Can you work these out from the model? Positions are in its coordinate system, mm. Face numbers are marked on the shaded views. A direction names the side the tool comes from. Give positions to 0.01 mm unless a question says otherwise; leave off trailing zeros. Write each loop counter-clockwise with the first axis right and the second up, starting at its lowest first coordinate (ties: lowest second). Pieces come first, ordered by that corner, then holes. Notation, with made-up numbers: (11.25, 77.25) - (69.25, 77.25) arc R15 cw to (69.25, 87.25) - close; hole circle Ø8 at (58, 0). An arc over 180 degrees is marked (long way). Use a Markdown table: item, result. Add a question column.
```python
from build123d import *

# Parameters (mm, degrees)
F2_W     = 460
F2_H     = 460
F2_W_2   = 420
F2_H_2   = 420
F3_DEPTH = 460
F4_R     = 5
F5_R     = 5


# Not quite as in the source:
# - the program builds the solid bodies; features that only make, move or delete a surface that nothing else refers to are left out


with BuildPart() as f3:
    # F2 (on Top) → F3 (new body)
    with BuildSketch(Plane.XY):
        Rectangle(F2_W, F2_H)
        Rectangle(F2_W_2, F2_H_2, mode=Mode.SUBTRACT)
    extrude(amount=F3_DEPTH)

    # F4
    f4_edges = [f3.edges().sort_by_distance(p)[0] for p in [
        (-230, 230, 230),
    ]]
    fillet(f4_edges, radius=F4_R)

    # F5
    f5_edges = [f3.edges().sort_by_distance(p)[0] for p in [
        (-230, -2.5, 460),
    ]]
    fillet(f5_edges, radius=F5_R)


solid = f3.part
```
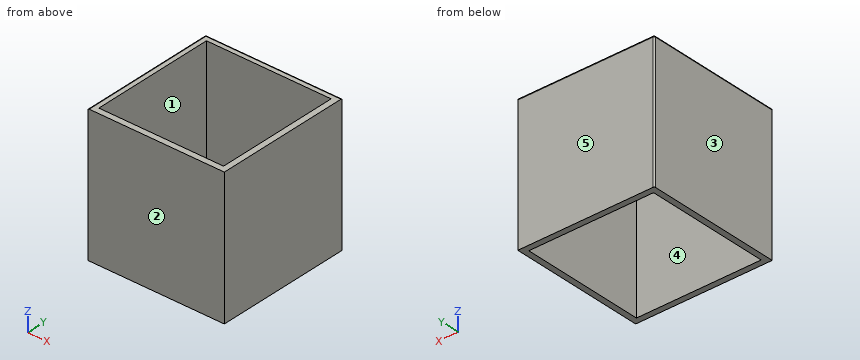
Q1. On a 3-axis mill with a long thin cutter (end or side, diameter ignored), from which of +Z, -Z, +X, -X, +Y, -Y can I reach the whole of each face in a straight line? I mean the marked faces 4 and 5. Say none if no direction works.
Q2. Suppose I cut it at C-C (y = -157.5). Please give me the cut outline in (x, z).
Q3. If I drill on probe 1 along Y at (x, z) = (-157.5, 179), over which ranges is the centre line in solid material (lowest first)? Write a range as [from, to].
Q4. Suppose I cut it at B-B (x = 30). Please give me the cut outline in (y, z), and give its area (3 significant figures).
Q5. If we mould it in two halves opening along X, with no side actions, what happens to the marked faces 1, 2 and 3? For each: released by +X, released by -X, zero draft, split by the parting line, or undercut.
Q6. Suppose I cut it at A-A (z = 232.5). Please give me the cut outline in (x, y).
Derived:
| question | item | result |
|---|---|---|
| 1 | face 4 | +Z, -Z |
| 1 | face 5 | +Z, -Z, +X, -X, +Y |
| 2 | outline | (-230, 0) - (-210, 0) - (-210, 460) - (-225, 460) arc R5 ccw to (-230, 455) - close; (210, 0) - (230, 0) - (230, 460) - (210, 460) - close |
| 3 | probe 1 | [-230, -210], [210, 230] |
| 4 | outline | (-230, 0) - (-210, 0) - (-210, 460) - (-230, 460) - close; (210, 0) - (230, 0) - (230, 455) arc R5 ccw to (225, 460) - (210, 460) - close |
| 4 | area | 18,400 mm² |
| 5 | face 1 | undercut |
| 5 | face 2 | zero draft |
| 5 | face 3 | released by -X |
| 6 | outline | (-230, -230) - (230, -230) - (230, 230) - (-225, 230) arc R5 ccw to (-230, 225) - close; hole (-210, -210) - (210, -210) - (210, 210) - (-210, 210) - close |
